The listing builds one solid part. Answer for the finished solid, in the listing's coordinates (mm). A direction names the side the tool comes from. Coordinates: 2 decimals unless noted, no trailing zeros. Order: outer loops, then holes, each group sorted by start corner. A loop starts at its lowest first (then second) coordinate and runs counter-clockwise, first axis right, second up. Notation, with made-up numbers: (-13, -17) -> (-7, -17) arc R29 cw to (-7, 4) -> close; hole circle Ø1 at (38.25, 80.5). An arc over 180 degrees is marked (long way). Return JSON: item names as keys, results as strings.
from build123d import *

# Parameters (mm, degrees)
SKETCH1_W           = 110
SKETCH1_H           = 280
BOSS_EXTRUDE1_DEPTH = 40
CUT_EXTRUDE2_DEPTH  = 124
SKETCH3_W           = 10.5
SKETCH3_H           = 5
CUT_EXTRUDE3_DEPTH  = 6
SKETCH4_W           = 10.5
SKETCH4_H           = 5
CUT_EXTRUDE4_DEPTH  = 6
CUT_EXTRUDE5_DEPTH  = 115
SKETCH6_W           = 5
SKETCH6_H           = 2.06188551
BOSS_EXTRUDE2_DEPTH = 10
SKETCH7_W           = 5
SKETCH7_H           = 2.339578052
BOSS_EXTRUDE3_DEPTH = 10
CUT_EXTRUDE6_DEPTH  = 128
SKETCH9_W           = 0.104698151
SKETCH9_H           = 1.212792293
CUT_EXTRUDE7_DEPTH  = 128
SKETCH10_W          = 100
SKETCH10_H          = 5
CUT_EXTRUDE9_DEPTH  = 128
SKETCH11_W          = 0.390083634
SKETCH11_H          = 4.996690545
CUT_EXTRUDE10_DEPTH = 128
SKETCH13_R          = 50
CUT_EXTRUDE11_DEPTH = 20
SKETCH14_W          = 10
SKETCH14_H          = 6.096695991
BOSS_EXTRUDE4_DEPTH = 10
SKETCH15_R          = 2
CUT_EXTRUDE12_DEPTH = 10


with BuildPart() as part:
    # Sketch1 → Boss-Extrude1 (new body)
    with BuildSketch(Plane(origin=(0, 0, 0), x_dir=(1, 0, 0), z_dir=(0, 1, 0))):
        with Locations((0, 71.043668932)):
            Rectangle(SKETCH1_W, SKETCH1_H)
        with BuildLine():
            Line((-44.5, -19.456331068), (-44.5, 161.543668932))
            ThreePointArc((-44.5, 161.543668932), (0, 206.043668932), (44.5, 161.543668932))
            Line((44.5, 161.543668932), (44.5, -19.456331068))
            ThreePointArc((44.5, -19.456331068), (0, -63.956331068), (-44.5, -19.456331068))
        make_face(mode=Mode.SUBTRACT)
    extrude(amount=BOSS_EXTRUDE1_DEPTH)

    # Sketch2 → Cut-Extrude2 (cut)
    with BuildSketch(Plane(origin=(55, 0, 0), x_dir=(0, 0, -1), z_dir=(1, 0, 0))):
        Polygon((116.043668932, 39.851089724), (36.043668932, 20), (35.922836705, 15.001460256), (116.043668932, 34.851089724), align=None)
    extrude(amount=-CUT_EXTRUDE2_DEPTH, mode=Mode.SUBTRACT)

    # Sketch3 → Cut-Extrude3 (cut)
    with BuildSketch(Plane(origin=(0, 40, 0), x_dir=(1, 0, 0), z_dir=(0, 1, 0))):
        with Locations((49.75, 118.535610254)):
            Rectangle(SKETCH3_W, SKETCH3_H)
    extrude(amount=-CUT_EXTRUDE3_DEPTH, mode=Mode.SUBTRACT)

    # Sketch4 → Cut-Extrude4 (cut)
    with BuildSketch(Plane(origin=(0, 40, 0), x_dir=(1, 0, 0), z_dir=(0, 1, 0))):
        with Locations((-49.75, 118.430912103)):
            Rectangle(SKETCH4_W, SKETCH4_H)
    extrude(amount=-CUT_EXTRUDE4_DEPTH, mode=Mode.SUBTRACT)

    # Sketch5 → Cut-Extrude5 (cut)
    with BuildSketch(Plane(origin=(55, 0, 0), x_dir=(0, 0, -1), z_dir=(1, 0, 0))):
        Polygon((116.035610254, 34.849093217), (136.82667534, 40), (116.035610254, 40), align=None)
    extrude(amount=-CUT_EXTRUDE5_DEPTH, mode=Mode.SUBTRACT)

    # Sketch6 → Boss-Extrude2 (add)
    with BuildSketch(Plane.ZY.offset(55)):
        with Locations((-118.430912103, 35.030942755)):
            Rectangle(SKETCH6_W, SKETCH6_H)
    extrude(amount=-BOSS_EXTRUDE2_DEPTH)

    # Sketch7 → Boss-Extrude3 (add)
    with BuildSketch(Plane(origin=(55, 0, 0), x_dir=(0, 0, -1), z_dir=(1, 0, 0))):
        with Locations((118.535610254, 35.169789026)):
            Rectangle(SKETCH7_W, SKETCH7_H)
    extrude(amount=-BOSS_EXTRUDE3_DEPTH)

    # Sketch8 → Cut-Extrude6 (cut)
    with BuildSketch(Plane(origin=(55, 0, 0), x_dir=(0, 0, -1), z_dir=(1, 0, 0))):
        Polygon((121.035610254, 36.087824076), (116.035610254, 34.849093217), (116.035610254, 36.339578052), (121.035610254, 36.339578052), align=None)
    extrude(amount=-CUT_EXTRUDE6_DEPTH, mode=Mode.SUBTRACT)

    # Sketch9 → Cut-Extrude7 (cut)
    with BuildSketch(Plane(origin=(-45, 0, 0), x_dir=(0, 0, -1), z_dir=(1, 0, 0))):
        with Locations((115.983261179, 35.455489364)):
            Rectangle(SKETCH9_W, SKETCH9_H)
    extrude(amount=-CUT_EXTRUDE7_DEPTH, mode=Mode.SUBTRACT)

    # Sketch10 → Cut-Extrude9 (cut)
    with BuildSketch(Plane(origin=(55, 0, 0), x_dir=(0, 0, -1), z_dir=(1, 0, 0))):
        with Locations((-14.346414702, 17.503309455)):
            Rectangle(SKETCH10_W, SKETCH10_H)
    extrude(amount=-CUT_EXTRUDE9_DEPTH, mode=Mode.SUBTRACT)

    # Sketch11 → Cut-Extrude10 (cut)
    with BuildSketch(Plane(origin=(55, 0, 0), x_dir=(0, 0, -1), z_dir=(1, 0, 0))):
        with Locations((35.848627115, 17.501654728)):
            Rectangle(SKETCH11_W, SKETCH11_H)
    extrude(amount=-CUT_EXTRUDE10_DEPTH, mode=Mode.SUBTRACT)

    # Sketch13 → Cut-Extrude11 (cut)
    with BuildSketch(Plane(origin=(0, 0, 0), x_dir=(-1, 0, 0), z_dir=(0, -1, 0))):
        with Locations((0, -14.346331068)):
            Circle(SKETCH13_R)
    extrude(amount=-CUT_EXTRUDE11_DEPTH, mode=Mode.SUBTRACT)

    # Sketch14 → Boss-Extrude4 (add)
    with BuildSketch(Plane.XY.offset(68.956331068)):
        with Locations((0, 36.951652005)):
            Rectangle(SKETCH14_W, SKETCH14_H)
    extrude(amount=BOSS_EXTRUDE4_DEPTH)

    # Sketch15 → Cut-Extrude12 (cut)
    with BuildSketch(Plane(origin=(0, 40, 0), x_dir=(1, 0, 0), z_dir=(0, 1, 0))):
        with Locations(Location((0, -73.956331068, 0), (0, 0, 270))):
            Circle(SKETCH15_R)
    extrude(amount=-CUT_EXTRUDE12_DEPTH, mode=Mode.SUBTRACT)


solid = part.part
1. The part is cut by section A-A on z = -17. Give the vertices of the cut face in (x, y), and give its area (3 significant figures).
Answer block:
{"outline": "(-55, 0) -> (-44.5, 0) -> (-44.5, 15) -> (-55, 15) -> close; (-55, 20) -> (-44.5, 20) -> (-44.5, 40) -> (-55, 40) -> close; (44.5, 0) -> (55, 0) -> (55, 15) -> (44.5, 15) -> close; (44.5, 20) -> (55, 20) -> (55, 40) -> (44.5, 40) -> close", "area": "735 mm2"}
2. The part is cut by section D-D on z = -150. Give the vertices of the cut face in (x, y).
Answer block:
{"outline": "(-55, 0) -> (-44.5, 0) -> (-44.5, 40) -> (-55, 40) -> close; (44.5, 0) -> (55, 0) -> (55, 40) -> (44.5, 40) -> close"}
3. The part is cut by section B-B on y = 6. Give the vertices of the cut face in (x, z), and give its area (3 significant figures).
Answer block:
{"outline": "(-55, -211.04) -> (55, -211.04) -> (55, 68.96) -> (-55, 68.96) -> close; hole (-44.5, -161.54) arc R44.5 ccw to (44.5, -161.54) -> (44.5, -8.45) arc R50 ccw (long way) to (-44.5, -8.45) -> close", "area": "7,940 mm2"}
4. For faces 1 (the face through (1.431, 7.397, 64.326)), 2 (the face through (-49.68, 24.79, -75.43)), 3 (the face through (44.5, 32, -34)), determine the directions among +Z, -Z, +X, -X, +Y, -Y from which every point of the face is accessible in a straight line to the end or side of a thin tool.
Answer block:
{"face 1": "-Y", "face 2": "+X, -X", "face 3": "+Y, -Y"}
5. This flat-tipped pin is pushed along its axis until it touches: pin 1 Ø1 at (x, y) = (43.5, 11) entering from +Z. Where does it stop, or does it pass through?
Answer block:
{"pin 1": "stops at z = 68.96"}
6. Consider line 1 (X direction, y = 37, z = -43); line 2 (Z direction, x = 0, y = 3); line 3 (Y direction, x = 38, z = 58). Determine where each line is inside the solid, lowest interval first. Write a range as from..to.
Answer block:
{"line 1": "x = -55..-44.5, 44.5..55", "line 2": "z = -211.04..-206.04, 64.35..68.96", "line 3": "y = 0..15, 20..40"}
7. The part is cut by section C-C on x = -23.5. Give the vertices of the cut face in (y, z).
Answer block:
{"outline": "(0, -211.04) -> (40, -211.04) -> (40, -199.33) -> (0, -199.33) -> close; (0, 58.48) -> (15, 58.48) -> (15, 64.35) -> (20, 64.35) -> (20, 57.25) -> (40, 57.25) -> (40, 68.96) -> (0, 68.96) -> close"}
8. Determine the mould class of faces 4 (the face through (-5, 37, 74)), 5 (the face through (49.824, 30.063, -76.6)), 6 (the face through (-0.979, 19.72, -206.033)), 7 (the face through (-44.5, 32, -32)) for opening direction X: pulls with the +X half, pulls with the -X half, needs draft (parallel to the pull), parting line crosses it, or undercut.
Answer block:
{"face 4": "pulls with the -X half", "face 5": "needs draft", "face 6": "undercut", "face 7": "undercut"}
